Can you work these out from the model? Positions are in its coordinate system, mm. Give positions to 0.01 mm unless a question says otherwise; leave off trailing zeros. Write each loop counter-clockwise with the first axis right and the second up, starting at its lowest first coordinate (ties: lowest second). Pieces come first, ordered by that corner, then holes. Notation, with made-up numbers: (26.25, 82.25) -> (66.25, 82.25) arc R20 ccw to (66.25, 92.25) -> close; hole circle Ø11 at (85.5, -25). An arc over 180 degrees is marked (long way). Answer as CSV lines item,"result". Start each with the question number.
1. If we section it at C-C on y = -10: Write out the boundary of the cut face in (x, z), plus the area to 3 significant figures.
2. I'm going to push flat-ended pins straight in: P1, Ø4, axis at y = 4.5, z = 26, coming from the -X side; P2, Ø2, axis at x = 2, y = -16, coming from the -Z side. Where does each tip first touch, or does it pass through?
3. If we section it at B-B on x = 2.75: Write out the boundary of the cut face in (y, z), plus the area to 4 significant figures.
4. I need wall thicknesses on line 1 (Y direction, x = 1.85, z = -30); line 2 (Z direction, x = 3.35, y = 17); line 3 (Z direction, x = 1.3, y = 14). Which ranges of each line are inside material? Lowest first, please. Write a range as [from, to].
5. If we section it at A-A on y = 0: Write out the boundary of the cut face in (x, z).
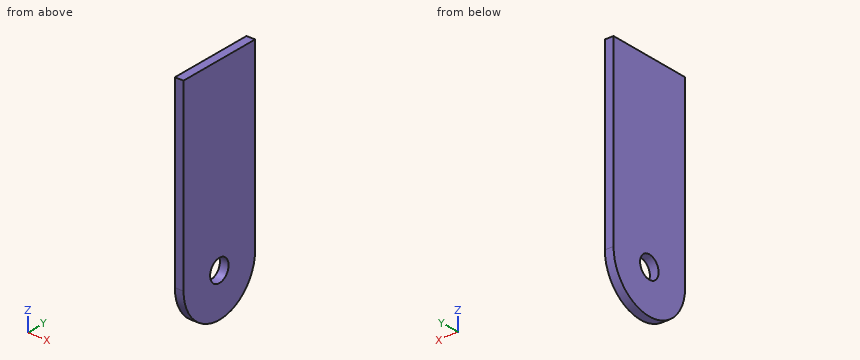
Autodesk Inventor part; units mm, degrees
ref_plane "YZ Plane" through (0, 0, 0) normal (1, 0, 0) x (0, 1, 0)
ref_plane "XZ Plane" through (0, 0, 0) normal (0, 1, 0) x (-1, 0, 0)
ref_plane "XY Plane" through (0, 0, 0) normal (0, 0, 1) x (1, 0, 0)
sketch "Sketch1" plane through (0, 0, 0) normal (1, 0, 0) x (0, 1, 0)
  line L0 (-20, -30) -> (20, -30)
  line L1 (20, -30) -> (20, 30)
  line L2 (20, 30) -> (-20, 30)
  line L3 (-20, 30) -> (-20, -30)
  line L4 (-20, -30) -> (20, 30) construction
  line L5 (20, -30) -> (-20, 30) construction
  circle A0 centre (0, -30) radius 20
  point P0 (0, 0)
  dimension "d0" = 40
  dimension "d1" = 60
extrude "Extrusion1" add sketch "Sketch1" along normal blind 4
sketch "Sketch4" plane through (4, 0, 0) normal (1, 0, 0) x (0, 0, -1)
  line L0 (-5, 20) -> (-55, 20)
  line L1 (-55, 20) -> (-55, -20)
  line L2 (-55, -20) -> (-5, -20)
  line L3 (-5, -20) -> (-5, 20)
  line L4 (-5, -104.205) -> (-5, 91.5035)
  line L5 (0, -143.3467) -> (0, 130.6452)
  line L6 (30, 20) -> (-30, 20)
  dimension "d40" = 50
  dimension "d41" = 40
  dimension "d49" = 5
  dimension "d50" = 0
  dimension "d52" = 0
extrude "Extrusion4" add sketch "Sketch4" against normal blind 4
sketch "Sketch2" plane through (0, 0, 0) normal (-1, 0, 0) x (0, 0, 1)
  arc A0 (-30, 20) -> (-30, -20) centre (-30, 0) ccw
  circle A1 centre (-30, 0) radius 5.15
  point P0 (0, 0)
  dimension "d4" = 10.3
extrude "Extrusion2" cut sketch "Sketch2" against normal blind 4
properties part number "houder"
Computed values:
1,outline,"(0, -47.32) -> (4, -47.32) -> (4, 55) -> (0, 55) -> close"
1,area,"409 mm2"
2,P1,"stops at x = 0"
2,P2,"stops at z = -43.23"
3,outline,"(-20, -30) arc R20 ccw to (20, -30) -> (20, 55) -> (-20, 55) -> close; hole circle Ø10.3 at (0, -30)"
3,area,"3,945 mm2"
4,line 1,"y = [-20, -5.15], [5.15, 20]"
4,line 2,"z = [-40.54, 55]"
4,line 3,"z = [-44.28, 55]"
5,outline,"(0, -50) -> (4, -50) -> (4, -35.15) -> (0, -35.15) -> close; (0, -24.85) -> (4, -24.85) -> (4, 55) -> (0, 55) -> close"
